Print and shaded views of the part. All mm, measured from the part's lowest x, y and z. Coordinates: 2 decimals unless noted, no trailing zeros. Order: outer loops, then holes, each group sorted by start corner. A loop starts at its lowest first (then second) coordinate and runs counter-clockwise, first axis right, second up. Notation, with made-up numbers: M 8.5,68.25 L 42.5,68.25 A23 ccw 42.5,99.25 Z; hole C 41.25,-39.75 d10. An arc over 180 degrees is marked long. Return JSON: item names as keys, results as strings.
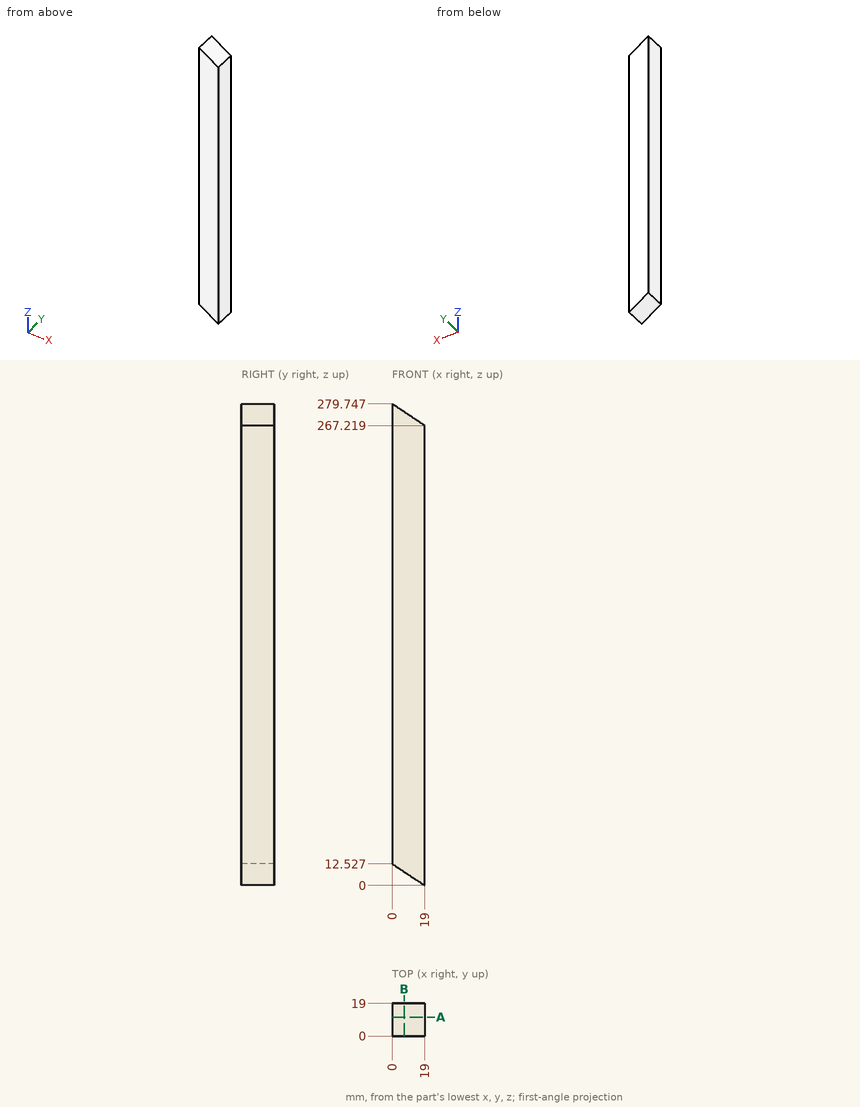
Item 1: Saw through at A-A (y = 11). Write the cut outline in (x, z), and give its area (3 significant figures).
Check result:
{"outline": "M 0,12.53 L 19,0 L 19,267.22 L 0,279.75 Z", "area": "5,080 mm2"}
Item 2: Saw through at B-B (x = 7). Write the cut outline in (y, z).
Check result:
{"outline": "M 0,7.91 L 19,7.91 L 19,275.13 L 0,275.13 Z"}
Item 3: Drop flat-ended pins along their axis: pin 1 Ø1.5 at (x, y) = (8, 15.5) entering from -Z; pin 2 Ø5 at (x, y) = (16.5, 14.5) entering from +Z (1 decimal); pin 3 Ø8 at (x, y) = (13, 12) entering from +Z. Give the stop position or say it passes through.
Check result:
{"pin 1": "stops at z = 6.76", "pin 2": "stops at z = 270.5", "pin 3": "stops at z = 273.81"}
Item 4: Wall check: line 1 (Z direction, x = 5, y = 12.5); line 2 (Z direction, x = 18, y = 16.75); line 3 (X direction, y = 8, z = 268.5) (1 decimal). Give the ranges that are in metal, low to high.
Check result:
{"line 1": "z = 9.23 to 276.45", "line 2": "z = 0.66 to 267.88", "line 3": "x = 0 to 17.1"}
